from build123d import *

# Parameters (mm, degrees)
F0_W     = 30
F0_H     = 50
F0_W_2   = 20
F0_H_2   = 40
F1_DEPTH = 5
F2_W     = 5
F2_H     = 4
F3_DEPTH = 6
F4_W     = 2
F4_H     = 2
F5_DEPTH = 20.11
F6_R     = 0.5
F7_R     = 0.7


with BuildPart() as f1:
    # F0 (on Top) → F1 (new body)
    with BuildSketch(Plane.XY):
        with Locations((15, 25)):
            Rectangle(F0_W, F0_H)
        with Locations((15, 25)):
            Rectangle(F0_W_2, F0_H_2, mode=Mode.SUBTRACT)
    extrude(amount=F1_DEPTH)

    # F2 (on face) → F3 (join)
    with BuildSketch(Plane.XY.offset(5)):
        with Locations((2.5, 27)):
            Rectangle(F2_W, F2_H)
        with Locations((27.5, 27)):
            Rectangle(F2_W, F2_H)
    extrude(amount=F3_DEPTH)

    # F4 (on face) → F5 (join)
    with BuildSketch(Plane(origin=(25, 0, 0), x_dir=(0, -1, 0), z_dir=(-1, 0, 0))):
        with Locations((-26, 1)):
            Rectangle(F4_W, F4_H)
    extrude(amount=F5_DEPTH)

    # F6
    f6_edges = [f1.edges().sort_by_distance(p)[0] for p in [
        (27.5, 29, 11),
        (27.5, 25, 11),
        (2.5, 25, 11),
        (2.5, 29, 11),
        (30, 0, 2.5),
        (25, 5, 2.5),
        (30, 50, 2.5),
        (0, 50, 2.5),
        (5, 45, 2.5),
        (5, 5, 2.5),
        (5, 27, 1),
        (5, 26, 2),
        (5, 25, 1),
        (25, 25, 1),
        (25, 26, 2),
        (25, 45, 2.5),
        (25, 27, 1),
        (0, 0, 2.5),
    ]]
    fillet(f6_edges, radius=F6_R)

    # F7
    f7_edges = [f1.edges().sort_by_distance(p)[0] for p in [
        (2.5, 25, 5),
        (27.5, 25, 5),
        (27.5, 29, 5),
        (2.5, 29, 5),
    ]]
    fillet(f7_edges, radius=F7_R)


solid = f1.part
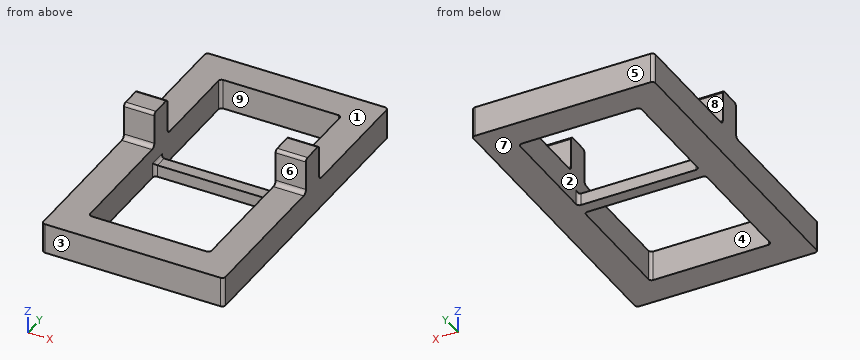
Can you work these out from the model? Positions are in its coordinate system, mm. Face numbers are marked on the shaded views. A direction names the side the tool comes from. Round coordinates to 2 decimals unless told otherwise and drop trailing zeros. Loops run counter-clockwise (first coordinate to the right, second up) from the corner with the lowest first, then second, coordinate; pieces in that order, holes last. Notation, with made-up numbers: (-5.75, 29.5) - (3.25, 29.5) arc R14 cw to (3.25, 35.5) - close; hole circle Ø5 at (38.5, 79). An arc over 180 degrees is marked (long way). Write item = value, one per line. Start each with the question number.
(1) For P1, Ø7.5, axis at x = 10, y = 8.5, coming from the +Z side; P2, Ø2.5, axis at x = 2, z = 8, coming from the -Y side; P3, Ø2, axis at y = 21.5, z = 7, coming from the +X side; P4, Ø1.6, axis at x = 16.5, y = 26, coming from the +Z side, each with a flat end and sliding along its axis, tell me the tip position at first contact or that it passes through.
(2) If we section it at B-B (x = 17.25): Please give me the cut outline in (y, z), and give its area (3 significant figures).
(3) If we section it at C-C (y = 38): Please give me the cut outline in (x, z).
(4) If I drill on probe 1 along Y at (x, z) = (12, 1.75); probe 2 along X at (y, z) = (34, 2.5); probe 3 along Y at (x, z) = (6.5, 3.25), over which ranges is the centre line in solid material (lowest first)? Write a range as [from, to].
(5) If we section it at A-A (z = 8.75): Please give me the cut outline in (x, y).
(6) If we mould it in two halves opening along Y, with no side actions, what happens to the marked faces 1, 2, 3 and 4? For each: released by +Y, released by -Y, zero draft, split by the parting line, or undercut.
(7) For the marked faces 5, 6, 7, 8 and 9, which set-ups out of +Z, -Z, +X, -X, +Y, -Y let a thin tool reach every point of the face, with its end or its side?
(8) If we section it at D-D (z = 4.5): Please give me the cut outline in (x, y).
Ans:
q1.P1 = 5
q1.P2 = 25
q1.P3 = through
q1.P4 = 2
q2.outline = (0, 0) - (5, 0) - (5, 5) - (0, 5) - close; (25, 0) - (27, 0) - (27, 2) - (25, 2) - close; (45, 0) - (50, 0) - (50, 5) - (45, 5) - close
q2.area = 54.0 mm²
q3.outline = (0, 0) - (5, 0) - (5, 5) - (0, 5) - close; (25, 0) - (30, 0) - (30, 5) - (25, 5) - close
q4.probe_1 = [0, 5], [25, 27], [45, 50]
q4.probe_2 = [0, 5], [25, 30]
q4.probe_3 = [0, 5], [45, 50]
q5.outline = (0, 25) - (5, 25) - (5, 29) - (0, 29) - close; (25, 25) - (30, 25) - (30, 29) - (25, 29) - close
q6.face_1 = zero draft
q6.face_2 = undercut
q6.face_3 = released by -Y
q6.face_4 = undercut
q7.face_5 = +Z, -Z, +X, -X, +Y
q7.face_6 = +Z, +X, -X, -Y
q7.face_7 = -Z, +X, -X, +Y, -Y
q7.face_8 = +Z, +X, -X, +Y
q7.face_9 = +Z, -Z
q8.outline = (0, 0.5) arc R0.5 ccw to (0.5, 0) - (29.5, 0) arc R0.5 ccw to (30, 0.5) - (30, 49.5) arc R0.5 ccw to (29.5, 50) - (0.5, 50) arc R0.5 ccw to (0, 49.5) - close; hole (5, 5.5) arc R0.5 ccw to (5.5, 5) - (24.5, 5) arc R0.5 ccw to (25, 5.5) - (25, 44.5) arc R0.5 ccw to (24.5, 45) - (5.5, 45) arc R0.5 ccw to (5, 44.5) - close
